Here's the drawing with two shaded views (mm, measured from the low corner). I have some questions. A direction names the side the tool comes from. Coordinates: 2 decimals unless noted, no trailing zeros. Write each loop counter-clockwise with the first axis right and the second up, starting at its lowest first coordinate (ties: lowest second). Pieces come first, ordered by that corner, then holes.
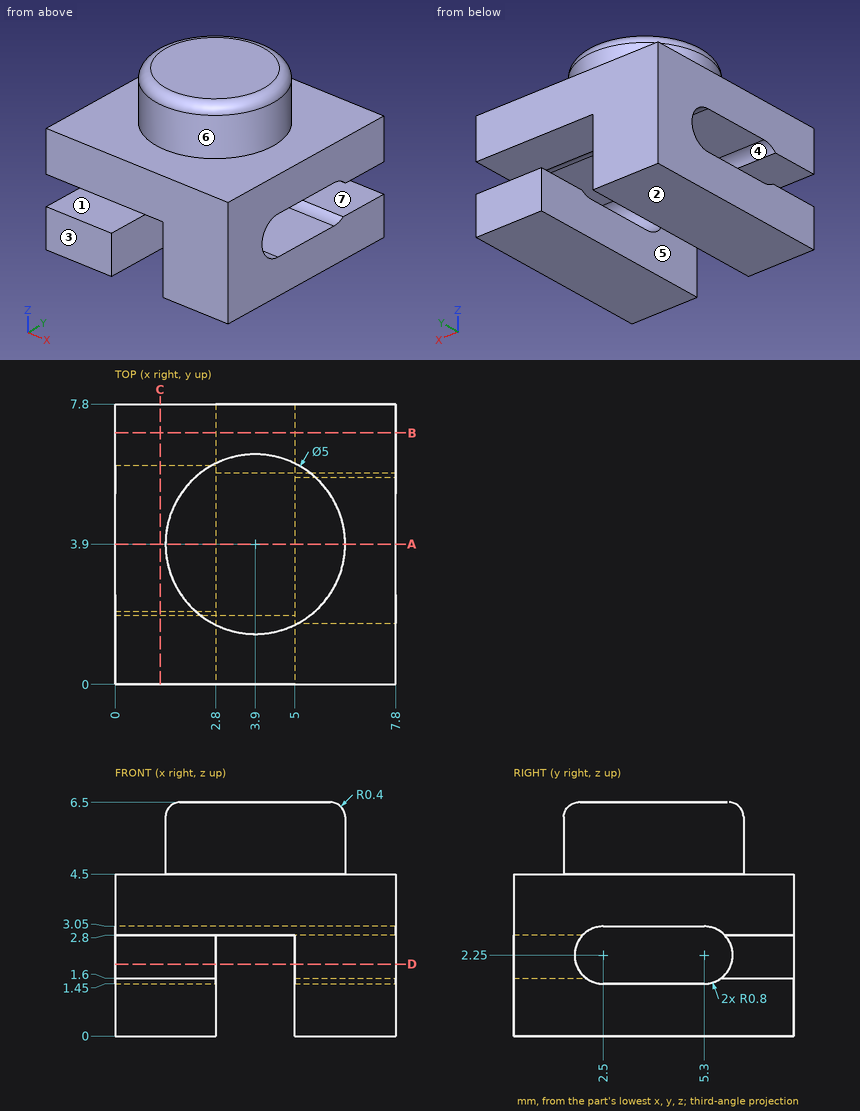
1. If we mould it in two halves opening along Z, with no side actions, what happens to the marked faces 1, 2 and 3? For each: pulls with the +Z half, pulls with the -Z half, needs draft (parallel to the pull), parting line crosses it, or undercut.
Verdict:
face 1: undercut
face 2: pulls with the -Z half
face 3: needs draft
2. On a 3-axis mill with a long thin cutter (end or side, diameter ignored), from which of +Z, -Z, +X, -X, +Y, -Y can I reach the whole of each face in a straight line? I mean the marked faces 4, 5, 6 and 7. Say none if no direction works.
Verdict:
face 4: +X, -X
face 5: -Z, +Y, -Y
face 6: +Z
face 7: +X, +Y
3. I want a section at B-B on y = 7. Please give me the cut outline in (x, z).
Verdict:
outline: (0, 0) - (2.8, 0) - (2.8, 2.8) - (7.8, 2.8) - (7.8, 4.5) - (0, 4.5) - close; (5, 0) - (7.8, 0) - (7.8, 1.6) - (5, 1.6) - close
4. Please list where these lines run through material, in increasing order: line 1 along Z through (x, y) = (7.75, 4.75); line 2 along Z through (x, y) = (5.5, 7); line 3 along X through (y, z) = (0.75, 1.5).
Verdict:
line 1: z = 0 to 1.45, 3.05 to 4.5
line 2: z = 0 to 1.6, 2.8 to 4.5
line 3: x = 0 to 2.8, 5 to 7.8
5. I want a section at D-D on z = 2. Please give me the cut outline in (x, y), plus the area to 3 significant figures.
Verdict:
outline: (0, 6.06) - (2.8, 6.06) - (2.8, 7.8) - (0, 7.8) - close; (5, 0) - (7.8, 0) - (7.8, 1.74) - (5, 1.74) - close
area: 9.74 mm2
6. I want a section at A-A on y = 3.9. Please give me the cut outline in (x, z), plus the area to 3 significant figures.
Verdict:
outline: (0, 0) - (2.8, 0) - (2.8, 1.45) - (0, 1.45) - close; (0, 3.05) - (7.8, 3.05) - (7.8, 4.5) - (6.4, 4.5) - (6.4, 6.1) arc R0.4 ccw to (6, 6.5) - (1.8, 6.5) arc R0.4 ccw to (1.4, 6.1) - (1.4, 4.5) - (0, 4.5) - close; (5, 0) - (7.8, 0) - (7.8, 1.45) - (5, 1.45) - close
area: 29.4 mm2
7. For pin 1 (2 mm diameter, centred on x = 4, z = 4.5, fed in from -Y); pin 2 (1.6 mm diameter, centred on x = 6, y = 6.5, fed in from +Z); pin 3 (1 mm diameter, centred on x = 4, y = 3.5, fed in from -Z), each with a flat end and sliding along its axis, tell me the tip position at first contact or that it passes through.
Verdict:
pin 1: stops at y = 0
pin 2: stops at z = 4.5
pin 3: stops at z = 3.05
8. I want a section at C-C on x = 1.25. Please give me the cut outline in (y, z), plus the area to 3 significant figures.
Verdict:
outline: (0, 0) - (7.8, 0) - (7.8, 4.5) - (0, 4.5) - (0, 2.8) - (1.92, 2.8) arc R0.8 cw to (2.5, 3.05) - (5.3, 3.05) arc R0.8 cw to (5.3, 1.45) - (2.5, 1.45) arc R0.8 cw to (2.03, 1.6) - (0, 1.6) - close
area: 26.5 mm2
